Model file for the job. Use its own axes, mm. A direction names the side the tool comes from. Coordinates: 2 decimals unless noted, no trailing zeros. Write each loop counter-clockwise with the first axis right and the second up, starting at its lowest first coordinate (ties: lowest second). Pieces come first, ordered by that corner, then holes. Notation, with made-up numbers: M 62,-21.5 L 82,-21.5 A26 ccw 82,-5.5 Z; hole C 59.5,-31 d6. An arc over 180 degrees is marked long. One line per question, with ' | ' between items. Start each with the question number.
(1) Cut at B-B (x = 35). Write the cut outline in (y, z).
(2) Tool access for faces 4 (the face through (36, 2, 3.112)), 5 (the face through (34.29, 2, -14)), 6 (the face through (36, 2, -15.05)), 7 (the face through (36, 2, -13.78)): list every direction of +Z, -Z, +X, -X, +Y, -Y with a clear straight run to the whole face (end or side of a thin tool).
(3) Cut at C-C (y = 0.7). Write the cut outline in (x, z) (1 decimal), plus the area to 3 significant figures.
(4) Wall check: probe 1 along Y at (x, z) = (5, -7.25); probe 2 along X at (y, z) = (1.15, -7) (3 decimals); probe 3 along X at (y, z) = (2.25, 2.25) (3 decimals). Give the ranges that are in metal, low to high.
(5) Cut at A-A (y = 2.3). Write the cut outline in (x, z) (1 decimal), plus the area to 3 significant figures.
(6) Cut at D-D (z = 1.5). Write the cut outline in (x, y) (1 decimal).
(7) Two-plate mould, pull along X, no slides. Class faces 1 (the face through (26, 1, -18.478)), 2 (the face through (34.29, 2.2, 2.5)), 3 (the face through (7.466, 1.431, -7.042)): +X half, -X half, draft (parallel to the pull), parting line (faces both ways), or undercut.
(8) Flat gauge pins, fed straight in: pin 1 Ø12.5 at (x, z) = (16, -9) entering from +Y; pin 2 Ø1 at (x, y) = (24.5, 2) entering from -Z; pin 3 Ø0.6 at (x, y) = (36, 2.5) entering from -Z; pin 4 Ø0.6 at (x, y) = (36.5, 2.5) entering from +Z. Where does each tip first touch, or does it go through?
Autodesk Inventor part; units mm, degrees
ref_plane "YZ Plane" through (0, 0, 0) normal (1, 0, 0) x (0, 1, 0)
ref_plane "XZ Plane" through (0, 0, 0) normal (0, 1, 0) x (-1, 0, 0)
ref_plane "XY Plane" through (0, 0, 0) normal (0, 0, 1) x (1, 0, 0)
sketch "Sketch1" plane through (0, 0, 0) normal (0, 1, 0) x (-1, 0, 0)
  line L0 (0, 0) -> (0, -11.938)
  line L1 (-15.24, 3.3655) -> (-15.24, -15.3035)
  line L2 (0, 0) -> (-15.24, 3.3655)
  line L3 (0, -11.938) -> (-15.24, -15.3035)
  line L4 (-15.24, 3.3655) -> (-19.05, 3.3655)
  line L5 (-19.05, 3.3655) -> (-19.05, 2.0955)
  line L6 (-19.05, 2.0955) -> (-15.24, 2.0955)
  line L7 (-15.24, 2.0955) -> (-15.24, 3.3655)
  line L8 (-15.24, -15.3035) -> (-19.05, -15.3035)
  line L9 (-19.05, -15.3035) -> (-19.05, -14.0335)
  line L10 (-19.05, -14.0335) -> (-15.24, -14.0335)
  line L11 (-15.24, -14.0335) -> (-15.24, -15.3035)
  line L12 (0, 0) -> (0, 3.175)
  line L13 (-15.24, 3.3655) -> (-15.24, 6.5405)
  line L14 (0, -11.938) -> (0, -15.113)
  line L15 (-15.24, -15.3035) -> (-15.24, -18.4785)
  line L16 (-15.24, -18.4785) -> (0, -15.113)
  line L17 (0, 3.175) -> (-15.24, 6.5405)
  line L18 (-15.24, 6.5405) -> (-34.29, 6.5405)
  line L19 (-19.05, 3.3655) -> (-34.29, 3.3655)
  line L20 (-34.29, 3.3655) -> (-34.29, 6.5405)
  line L21 (-15.24, -18.4785) -> (-34.29, -18.4785)
  line L22 (-34.29, -18.4785) -> (-34.29, -15.3035)
  line L23 (-34.29, -15.3035) -> (-19.05, -15.3035)
  line L24 (-34.29, 6.5405) -> (-37.465, 6.5405)
  line L25 (-37.465, 6.5405) -> (-37.465, -18.4785)
  line L26 (-37.465, -18.4785) -> (-34.29, -18.4785)
  line L27 (-34.29, -18.4785) -> (-34.29, 6.5405)
  line L28 (-15.24, -15.3035) -> (-34.29, -15.3035)
  line L29 (-34.29, -15.3035) -> (-34.29, 3.3655)
  line L30 (-34.29, 3.3655) -> (-15.24, 3.3655)
  line L31 (-15.24, 3.3655) -> (-15.24, -15.3035)
  line L32 (-15.24, 3.3655) -> (-34.29, 3.3655)
  line L33 (-34.29, 3.3655) -> (-34.29, 6.5405)
  line L34 (-34.29, 6.5405) -> (-15.24, 6.5405)
  line L35 (-15.24, 6.5405) -> (-15.24, 3.3655)
  dimension "d0" = 11.938
  dimension "d1" = 15.24
  dimension "d2" = 18.669
  dimension "d3" = 3.3655
  dimension "d4" = 3.81
  dimension "d5" = 1.27
  dimension "d6" = 3.81
  dimension "d7" = 1.27
  dimension "d8" = 3.175
  dimension "d9" = 3.175
  dimension "d10" = 3.175
  dimension "d11" = 3.175
  dimension "d12" = 19.05
  dimension "d13" = 3.175
extrude "Extrusion4" add sketch "Sketch1" along normal blind 1.5875
sketch "Sketch4" plane through (0, 1.5875, 0) normal (0, 1, 0) x (1, 0, 0)
  circle A0 centre (8.636, 5.969) radius 1.5875
  line L0 (0, 15.113) -> (0, -3.175)
  point P0 (0, 0)
  dimension "d26" = 3.175
  dimension "d27" = 8.636
extrude "Extrusion5" cut sketch "Sketch4" against normal blind 1.5875
chamfer "Chamfer2" distance 1.27 angle 45 1 edges at (7.0485, 0, -5.969)
sketch "Sketch5" plane through (0, 1.5875, 0) normal (0, 1, 0) x (1, 0, 0)
  circle A0 centre (8.636, 5.969) radius 1.5875
  line L0 (0, 15.113) -> (0, -3.175)
  line L1 (0, -3.175) -> (15.24, -6.5405)
  line L2 (15.24, -6.5405) -> (37.465, -6.5405)
  line L3 (37.465, -6.5405) -> (37.465, 18.4785)
  line L4 (37.465, 18.4785) -> (15.24, 18.4785)
  line L5 (15.24, 18.4785) -> (0, 15.113)
  line L6 (37.465, 15.0495) -> (34.29, 15.0495)
  line L7 (34.29, 15.0495) -> (34.29, 13.7795)
  line L8 (34.29, 13.7795) -> (37.465, 13.7795)
  line L9 (37.465, 13.7795) -> (37.465, 15.0495)
  line L10 (37.465, -3.1115) -> (34.29, -3.1115)
  line L11 (34.29, -3.1115) -> (34.29, -1.8967)
  line L12 (34.29, -1.8967) -> (37.465, -1.8967)
  line L13 (37.465, -1.8967) -> (37.465, -3.1115)
  line L14 (15.24, -6.5405) -> (37.465, -6.5405)
  line L15 (37.465, -6.5405) -> (37.465, -3.1115) construction
  line L16 (37.465, 18.4785) -> (15.24, 18.4785) construction
  line L17 (37.465, 15.0495) -> (37.465, 18.4785) construction
  point P0 (0, 0)
  dimension "d36" = 3.429
  dimension "d37" = 1.27
  dimension "d38" = 3.175
extrude "Extrusion6" add sketch "Sketch5" along normal blind 1.27 contours L3 L8 L7 L6 | L10 L11 L12 L3
equation "\"d3\" = -0.5 * d0 + 0.5 * d2"
properties part number "phototransistorMount2" material "ABS Plastic"
Filled in:
1) outline: M 0,-18.48 L 1.59,-18.48 L 1.59,-15.05 L 2.86,-15.05 L 2.86,-13.78 L 1.59,-13.78 L 1.59,1.9 L 2.86,1.9 L 2.86,3.11 L 1.59,3.11 L 1.59,6.54 L 0,6.54 Z
2) face 4: +Z, +X, -X, +Y | face 5: +Z, -Z, -X, +Y | face 6: -Z, +X, -X, +Y | face 7: +X, -X, +Y
3) outline: M 0,-15.1 L 15.2,-18.5 L 37.5,-18.5 L 37.5,6.5 L 15.2,6.5 L 0,3.2 Z; hole C 8.6,-6 d4.3 | area: 871 mm²
4) probe 1: 0 to 1.59 | probe 2: 0 to 7.275, 9.997 to 37.465 | probe 3: 34.29 to 37.465
5) outline: M 34.3,-15 L 37.5,-15 L 37.5,-13.8 L 34.3,-13.8 Z; M 34.3,1.9 L 37.5,1.9 L 37.5,3.1 L 34.3,3.1 Z | area: 7.89 mm²
6) outline: M 0,0 L 37.5,0 L 37.5,1.6 L 0,1.6 Z
7) face 1: draft | face 2: -X half | face 3: undercut
8) pin 1: y = 1.59 | pin 2: z = -18.48 | pin 3: z = -15.05 | pin 4: z = 3.11
